Design review of the part built by this model. Coordinates are the model's own, in mm. A direction names the side the tool comes from. Coordinates: 2 decimals unless noted, no trailing zeros. Loops run counter-clockwise (first coordinate to the right, second up) from the corner with the lowest first, then second, coordinate; pieces in that order, holes last. Notation, with made-up numbers: (5.25, -11) - (60.25, -11) arc R18 cw to (60.25, 2) - close; hole circle Ø1 at (-2.75, -39). An arc over 180 degrees is marked (long way). Answer in a Markdown table with one row per item. Add a question column.
(1) The part is to be moulded in two halves that separate along X. For faces 6 (the face through (14.217, 2, 13)), 7 (the face through (-3, 1.907, 13)), 8 (the face through (-16.383, 2.3, 12.8)), 9 (the face through (-19, 1.131, 13)), say which applies: released by +X, released by -X, zero draft, split by the parting line, or undercut.
(2) To check wall thickness, follow L1, parallel to Z at x = -5, y = 1.55; L2, parallel to Y at x = 0, z = 19.75; L3, parallel to Y at x = -18.5, z = 17.25. State the ranges of each line that lie inside material, in increasing order. Write a range as [from, to].
(3) We need section A-A, the plane x = -15. Write out the cut boundary in (y, z).
(4) Clearance check with flat-ended pins moving along their axes: pin 1 (4 mm diameter, centred on x = -18.5, z = 13.5, fed in from +Y); pin 2 (0.6 mm diameter, centred on y = 0, z = 17, fed in from -X); pin 3 (6 mm diameter, centred on x = -4.5, z = 15, fed in from +Y). State where each tip first meets the part, or that it passes through.
(5) For faces 1 (the face through (12, 0.762, 13)), 2 (the face through (13.117, 2.07, -0.761)), 3 (the face through (13.117, 2.07, 26.74)), 4 (the face through (-16.883, 0, 13)), 5 (the face through (-18, 2.733, 13)), list the 3-axis set-ups (+Z, -Z, +X, -X, +Y, -Y) from which the entire face can be reached by the end or side of a thin tool; tool diameter is ignored.
(6) We need section B-B, the plane y = -0.3. Write out the cut boundary in (x, z).
from build123d import *

# Parameters (mm, degrees)
BOSS_EXTRUDE3_DEPTH = 26
FILLET6_DEPTH       = 26
SKETCH6_R           = 0.5
BOSS_EXTRUDE6_DEPTH = 1.5
LPATTERN1_COUNT     = 2
LPATTERN1_PITCH     = 27.5


with BuildPart() as part:
    # Sketch4 → Boss-Extrude3 (new body)
    with BuildSketch(Plane.XY):
        with BuildLine():
            Line((-16.882676832, -0.738323828), (9.917323168, -0.738323828))
            Line((9.917323168, -0.738323828), (9.917323168, 0.761676172))
            Line((9.917323168, 0.761676172), (14.217323168, 0.761676172))
            Line((14.217323168, 0.761676172), (14.217323168, 3.761676172))
            Line((14.217323168, 3.761676172), (10.417323168, 3.761676172))
            Line((10.417323168, 3.761676172), (10.417323168, 1.907320096))
            Line((10.417323168, 1.907320096), (-16.382676832, 1.907320096))
            Line((-16.382676832, 1.907320096), (-16.382676832, 2.732812963))
            Line((-16.382676832, 2.732812963), (-19.929938074, 2.732812963))
            ThreePointArc((-19.929938074, 2.732812963), (-21.061793852, 2.121559656), (-21.882676832, 1.131166179))
            Line((-21.882676832, 1.131166179), (-16.882676832, 1.131166179))
            Line((-16.882676832, 1.131166179), (-16.882676832, -0.738323828))
        make_face()
    extrude(amount=BOSS_EXTRUDE3_DEPTH)

    # Fillet6: read off the stored shape, not the designer's step
    # Fillet6 outline → Fillet6 (cut)
    with BuildSketch(Plane.XY):
        with BuildLine():
            Line((10.417323168, 3.761676172), (10.417323168, 1.907320096))
            add(Edge.make_bspline(
                [(10.417323168, 1.907320096), (10.684335221, 2.237350554), (10.951347275, 2.567381012), (11.617088855, 3.247333717), (12.422778443, 3.640500924), (13.36841604, 3.74688263), (13.792869604, 3.754279401), (14.217323168, 3.761676172)],
                knots=[0, 0, 0, 0, 0, 0, 0.5, 0.5, 1, 1, 1, 1, 1, 1], degree=5))
            Line((14.217323168, 3.761676172), (10.417323168, 3.761676172))
        make_face()
    extrude(amount=FILLET6_DEPTH, mode=Mode.SUBTRACT)

    # Sketch6 → Boss-Extrude6 (add)
    with BuildSketch(Plane.XY.offset(26)):
        with Locations(Location((12.617323168, 2.091676172, 0), (0, 0, 180))):
            Circle(SKETCH6_R)
    boss_extrude6 = extrude(amount=BOSS_EXTRUDE6_DEPTH)

    # LPattern1: Boss-Extrude6 ×2
    with Locations(*[(0, 0, -i * LPATTERN1_PITCH) for i in range(1, LPATTERN1_COUNT)]):
        add(boss_extrude6)


solid = part.part
Responses:
| question | item | result |
|---|---|---|
| 1 | face 6 | released by +X |
| 1 | face 7 | undercut |
| 1 | face 8 | undercut |
| 1 | face 9 | zero draft |
| 2 | L1 | z = [0, 26] |
| 2 | L2 | y = [-0.74, 1.91] |
| 2 | L3 | y = [1.13, 2.73] |
| 3 | outline | (-0.74, 0) - (1.91, 0) - (1.91, 26) - (-0.74, 26) - close |
| 4 | pin 1 | stops at y = 2.73 |
| 4 | pin 2 | stops at x = -16.88 |
| 4 | pin 3 | stops at y = 1.91 |
| 5 | face 1 | +Z, -Z, +X, -Y |
| 5 | face 2 | -Z |
| 5 | face 3 | +Z |
| 5 | face 4 | +Z, -Z, -X, -Y |
| 5 | face 5 | +Z, -Z, -X, +Y |
| 6 | outline | (-16.88, 0) - (9.92, 0) - (9.92, 26) - (-16.88, 26) - close |
